For this review, use the dimensioned drawing (mm, ordinates from the lowest corner) and the shaded views. A direction names the side the tool comes from. Round coordinates to 2 decimals unless told otherwise and drop trailing zeros. Loops run counter-clockwise (first coordinate to the right, second up) from the corner with the lowest first, then second, coordinate; pieces in that order, holes last. Notation, with made-up numbers: M -15,73 L -1,73 A26 ccw -1,94 Z; hole C -23.75,10.25 d11. An arc over 180 degrees is marked long. One line per item, written item: value. Start each with the question number.
Item 1: We need section B-B (y = 3.5). Write out the cut boundary in (x, z).
Item 2: We need section D-D (z = 17.75). Write out the cut boundary in (x, y).
Item 3: For the marked faces 5, 6 and 7, list the 3-axis set-ups (+Z, -Z, +X, -X, +Y, -Y) from which the entire face can be reached by the end or side of a thin tool; tool diameter is ignored.
Item 4: Clearance check with flat-ended pins moving along their axes: pin 1 (1 mm diameter, centred on y = 6.5, z = 15.5, fed in from -X); pin 2 (2.5 mm diameter, centred on y = 5, z = 11, fed in from -X); pin 3 (1 mm diameter, centred on x = 5, y = 11, fed in from +Z); pin 4 (1 mm diameter, centred on x = 8, z = 4, fed in from +Y). State where each tip first meets the part, or that it passes through.
Item 5: For line 1 along Y through (x, z) = (3, 11); line 2 along Y through (x, z) = (6.75, 19.5); line 3 along Z through (x, y) = (4.25, 10.25), list the stretches that pass through material, from the lowest coordinate up.
Item 6: We need section A-A (z = 10.5). Write out the cut boundary in (x, y).
Item 7: Mouldability with a two-part tool opening along Z and no side actions: class the marked faces 1, 2, 3 and 4 as released by +Z, released by -Z, zero draft, split by the parting line, or undercut.
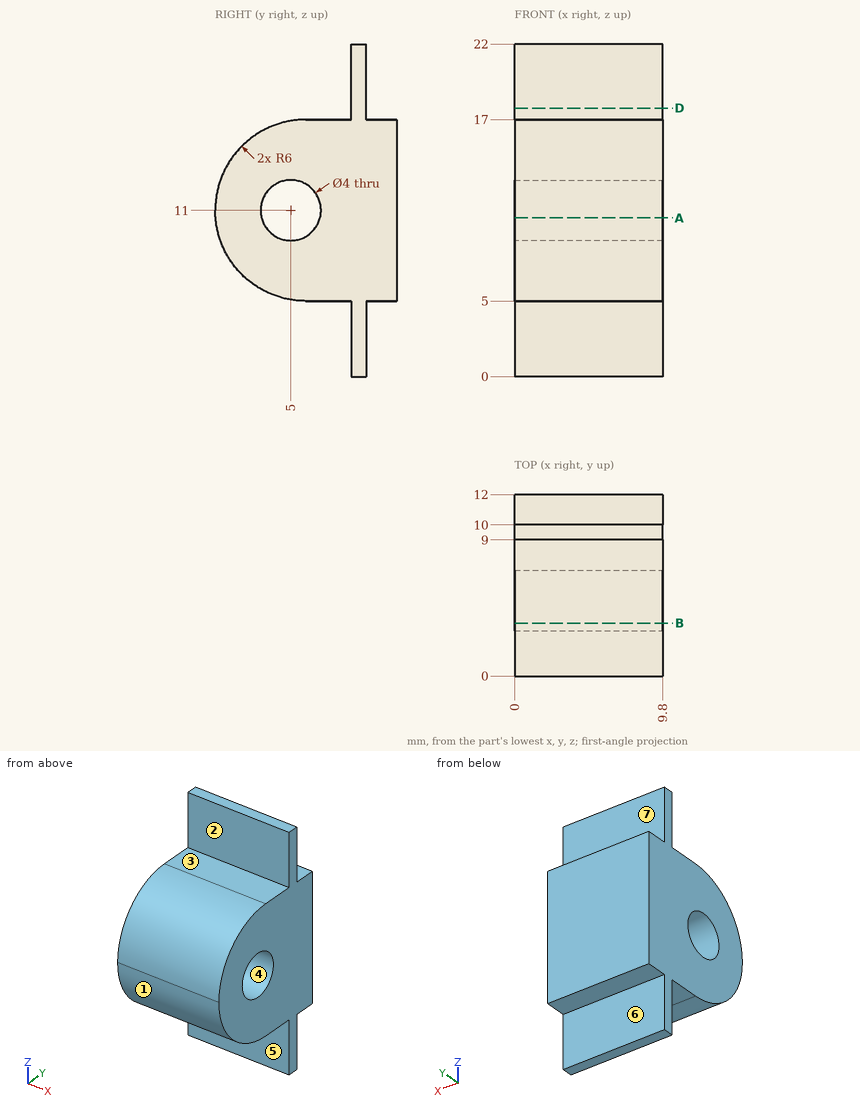
A:
1. outline: M 0,5.55 L 9.8,5.55 L 9.8,9.68 L 0,9.68 Z; M 0,12.32 L 9.8,12.32 L 9.8,16.45 L 0,16.45 Z
2. outline: M 0,9 L 9.8,9 L 9.8,10 L 0,10 Z
3. face 5: -Z, +X, -X, -Y
3. face 6: -Z, +X, -X, +Y
3. face 7: +Z, +X, -X, +Y
4. pin 1: x = 0
4. pin 2: through
4. pin 3: z = 17
4. pin 4: y = 10
5. line 1: 0 to 3, 7 to 12
5. line 2: 9 to 10
5. line 3: 5 to 17
6. outline: M 0,0.02 L 9.8,0.02 L 9.8,3.06 L 0,3.06 Z; M 0,6.94 L 9.8,6.94 L 9.8,12 L 0,12 Z
7. face 1: released by -Z
7. face 2: zero draft
7. face 3: released by +Z
7. face 4: undercut
